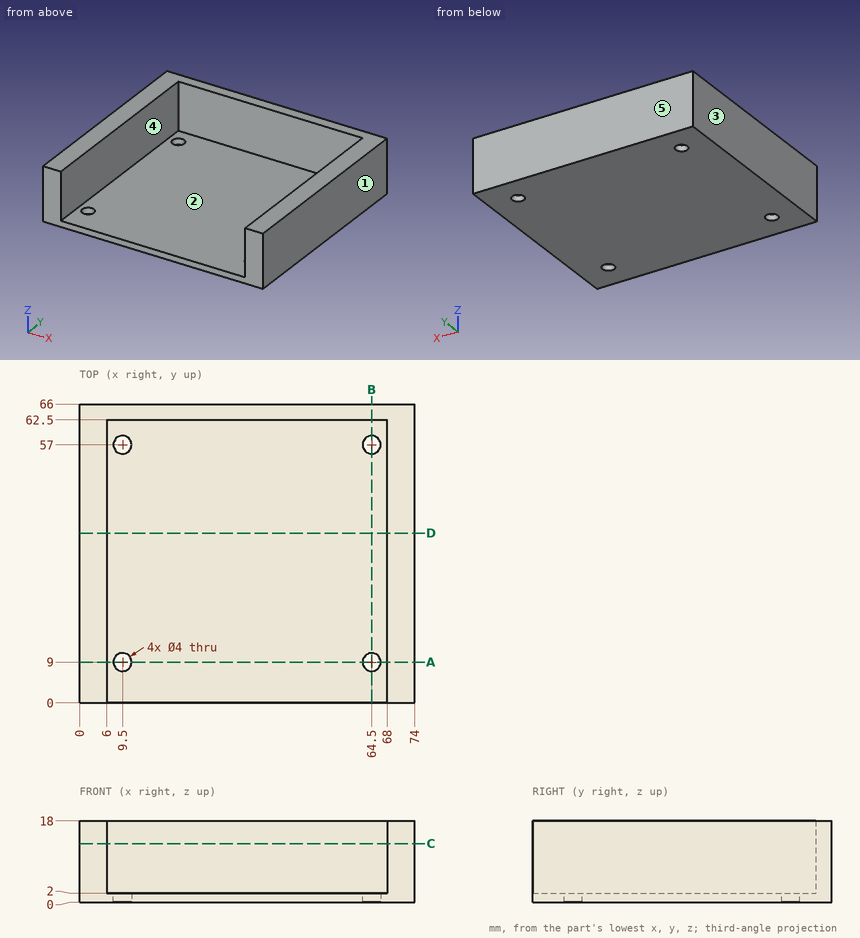
Can you work these out from the drawing? Everything is in mm from the part's minimum corner. A direction names the side the tool comes from. Coordinates: 2 decimals unless noted, no trailing zeros. Loops run counter-clockwise (first coordinate to the right, second up) from the corner with the lowest first, then second, coordinate; pieces in that order, holes last.
1) Imagine slicing it at A-A on y = 9. List the corners of the cut face in (x, z) for me, plus the area to 3 significant figures.
2) Imagine slicing it at B-B on x = 64.5. List the corners of the cut face in (y, z) for me, plus the area to 3 significant figures.
3) Imagine slicing it at D-D on y = 37.5. List the corners of the cut face in (x, z) for me.
4) Which directions (+Z, -Z, +X, -X, +Y, -Y) give clear straight access to the entire face, cutting with the end or side of a thin tool? Please do the marked faces 1 and 2.
5) Thinking about a two-plate mould opening in X: for the marked faces 3, 4 and 5, which applies, pulls with the +X half, pulls with the -X half, needs draft (parallel to the pull), parting line crosses it, or undercut?
6) For pin 1 (1.5 mm diameter, centred on x = 63.5, z = 8.5, fed in from -Y); pin 2 (3 mm diameter, centred on x = 64.5, y = 57, fed in from -Z); pin 3 (2 mm diameter, centred on x = 65, y = 8, fed in from +Z), each with a flat end and sliding along its axis, tell me the tip position at first contact or that it passes through.
7) Imagine slicing it at C-C on z = 13. List the corners of the cut face in (x, y) for me.
8) I need wall thicknesses on probe 1 along Y at (x, z) = (9.5, 0.4); probe 2 along X at (y, z) = (34, 3); probe 3 along Z at (x, y) = (41.5, 59.5). Which ranges of each line are inside material? Lowest first, please.
Completed:
1. outline: (0, 0) - (7.5, 0) - (7.5, 2) - (6, 2) - (6, 18) - (0, 18) - close; (11.5, 0) - (62.5, 0) - (62.5, 2) - (11.5, 2) - close; (66.5, 0) - (74, 0) - (74, 18) - (68, 18) - (68, 2) - (66.5, 2) - close
1. area: 324 mm2
2. outline: (0, 0) - (7, 0) - (7, 2) - (0, 2) - close; (11, 0) - (55, 0) - (55, 2) - (11, 2) - close; (59, 0) - (66, 0) - (66, 18) - (62.5, 18) - (62.5, 2) - (59, 2) - close
2. area: 172 mm2
3. outline: (0, 0) - (74, 0) - (74, 18) - (68, 18) - (68, 2) - (6, 2) - (6, 18) - (0, 18) - close
4. face 1: +Z, -Z, +X, +Y, -Y
4. face 2: +Z, -Y
5. face 3: pulls with the -X half
5. face 4: undercut
5. face 5: needs draft
6. pin 1: stops at y = 62.5
6. pin 2: passes through
6. pin 3: stops at z = 2
7. outline: (0, 0) - (6, 0) - (6, 62.5) - (68, 62.5) - (68, 0) - (74, 0) - (74, 66) - (0, 66) - close
8. probe 1: y = 0 to 7, 11 to 55, 59 to 66
8. probe 2: x = 0 to 6, 68 to 74
8. probe 3: z = 0 to 2
